Part print with two shaded views. Sizes in mm from the minimum x, y, z corner. A direction names the side the tool comes from. Round coordinates to 2 decimals unless told otherwise and drop trailing zeros. Write each loop counter-clockwise with the first axis right and the second up, starting at its lowest first coordinate (ties: lowest second). Pieces come first, ordered by that corner, then holes. Notation, with made-up numbers: (25, 45) -> (77, 45) arc R16 cw to (77, 53) -> close; hole circle Ø1 at (-37.5, -31). An arc over 180 degrees is marked (long way). Answer as CSV lines item,"result".
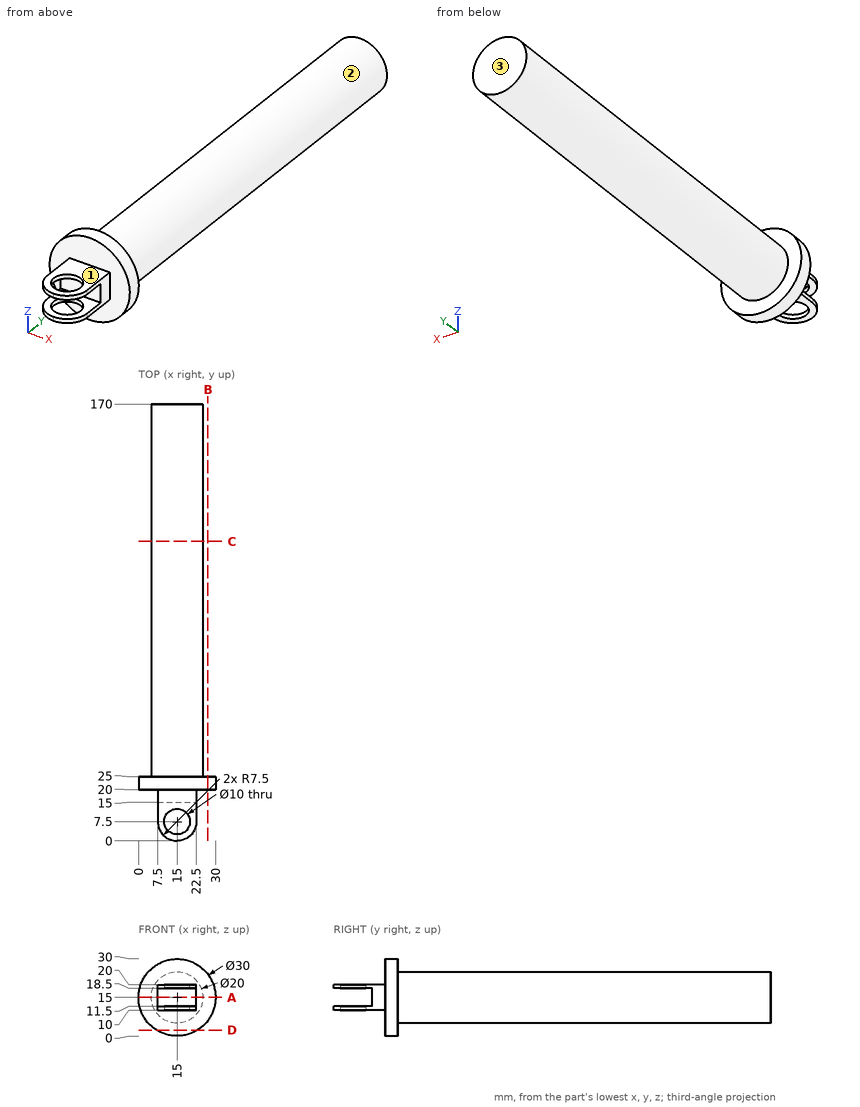
1. Which spindle directions (+Z, -Z, +X, -X, +Y, -Y) get a long thin tool onto all of the face, cutting with end or side? Do the marked faces 1, 2 and 3. Say none if no direction does.
Results found:
face 1,"+Z, +X, -X, -Y"
face 2,"+Y"
face 3,"+Z, -Z, +X, -X, +Y"
2. Cut at A-A, the plane z = 15. Write the cut outline in (x, y), then the cut area to 4 significant figures.
Results found:
outline,"(0, 20) -> (7.5, 20) -> (7.5, 15) -> (22.5, 15) -> (22.5, 20) -> (30, 20) -> (30, 25) -> (25, 25) -> (25, 170) -> (5, 170) -> (5, 25) -> (0, 25) -> close"
area,"3,125 mm2"
3. Cut at B-B, the plane x = 27. Write the cut outline in (y, z), then the cut area to 3 significant figures.
Results found:
outline,"(20, 6) -> (25, 6) -> (25, 24) -> (20, 24) -> close"
area,"90.0 mm2"
4. Cut at D-D, the plane z = 2.25. Write the cut outline in (x, y), then the cut area to 3 significant figures.
Results found:
outline,"(7.1, 20) -> (22.9, 20) -> (22.9, 25) -> (7.1, 25) -> close"
area,"79.0 mm2"
5. Probe line 1 along Y through (x, z) = (15, 18.8); line 2 along X through (y, z) = (7.5, 11.2); line 3 along Y through (x, z) = (13.5, 11.25). List the from-to ranges inside material, lowest first.
Results found:
line 1,"y = 0 to 2.5, 12.5 to 170"
line 2,"x = 7.5 to 10, 20 to 22.5"
line 3,"y = 0.15 to 2.73, 12.27 to 170"
6. Drop flat-ended pins along their axis: pin 1 Ø3 at (x, z) = (8, 20) entering from -Y; pin 2 Ø5 at (y, z) = (84, 9) entering from -X; pin 3 Ø8 at (y, z) = (14, 12.5) entering from +X; pin 4 Ø15 at (x, z) = (19.5, 12) entering from -Y. Give the stop position or say it passes through.
Results found:
pin 1,"stops at y = 2.4"
pin 2,"stops at x = 5.63"
pin 3,"stops at x = 22.5"
pin 4,"stops at y = 0"
7. Cut at C-C, the plane y = 116.5. Write the cut outline in (x, z), then the cut area to 3 significant figures.
Results found:
outline,"circle Ø20 at (15, 15)"
area,"314 mm2"
